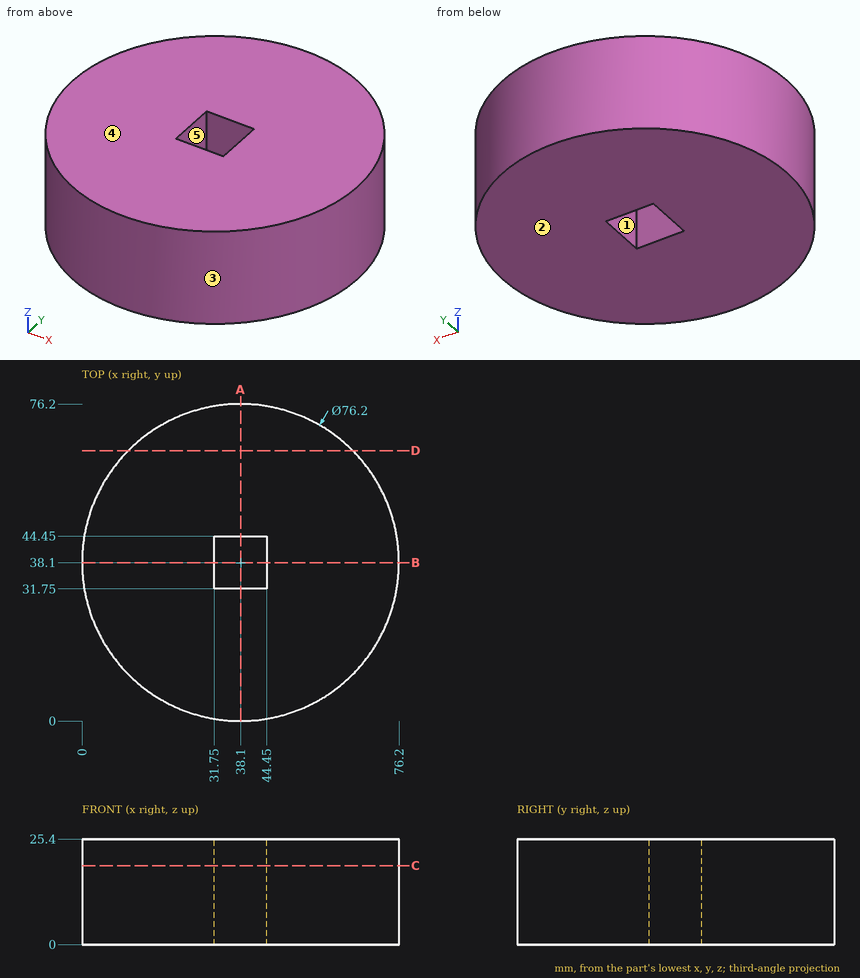
The figure shows three views and two pictorial views of one solid part (mm, origin at its lowest corner). Answer the questions. A direction names the side the tool comes from. Coordinates: 2 decimals unless noted, no trailing zeros. Write each loop counter-clockwise with the first axis right and the second up, starting at its lowest first coordinate (ties: lowest second). Pieces come first, ordered by that corner, then holes.
1. Flat-ended cylindrical pins translate along their axes: pin 1 (6.5 mm diameter, centred on x = 39.5, z = 17, fed in from +Y); pin 2 (10 mm diameter, centred on x = 39.5, z = 15.5, fed in from -Y); pin 3 (1 mm diameter, centred on x = 58, z = 8.5, fed in from -Y). Find the tip coordinate at first contact, or state that the pin passes through.
Results list:
pin 1: stops at y = 76.2
pin 2: stops at y = 0
pin 3: stops at y = 5.31
2. Consider line 1 along X through (y, z) = (39, 4.25); line 2 along Y through (x, z) = (33, 17.5); line 3 along Y through (x, z) = (42, 23.75). Determine where each line is inside the solid, lowest interval first.
Results list:
line 1: x = 0.01 to 31.75, 44.45 to 76.19
line 2: y = 0.34 to 31.75, 44.45 to 75.86
line 3: y = 0.2 to 31.75, 44.45 to 76
3. For the marked faces 1 and 2, determine the directions among +Z, -Z, +X, -X, +Y, -Y from which every point of the face is accessible in a straight line to the end or side of a thin tool.
Results list:
face 1: +Z, -Z
face 2: -Z, +X, -X, +Y, -Y
4. The part is cut by section C-C, the plane z = 19. Write down the section's boundary in (x, y).
Results list:
outline: circle Ø76.2 at (38.1, 38.1); hole (31.75, 31.75) - (44.45, 31.75) - (44.45, 44.45) - (31.75, 44.45) - close
5. For a pull along Y with two mould halves and no side action, classify the marked faces 3, 4 and 5 as +Y half, -Y half, draft (parallel to the pull), parting line (faces both ways), or undercut.
Results list:
face 3: parting line
face 4: draft
face 5: undercut
6. The part is cut by section A-A, the plane x = 38.1. Write down the section's boundary in (y, z).
Results list:
outline: (0, 0) - (31.75, 0) - (31.75, 25.4) - (0, 25.4) - close; (44.45, 0) - (76.2, 0) - (76.2, 25.4) - (44.45, 25.4) - close
7. The part is cut by section D-D, the plane y = 65. Write down the section's boundary in (x, z).
Results list:
outline: (11.12, 0) - (65.08, 0) - (65.08, 25.4) - (11.12, 25.4) - close
